Verification items for the finished model (mm, model axes). A direction names the side the tool comes from. Coordinates: 2 decimals unless noted, no trailing zeros. Order: outer loops, then holes, each group sorted by start corner. A loop starts at its lowest first (then second) coordinate and runs counter-clockwise, first axis right, second up. Notation, with made-up numbers: (-4.5, 71) -> (49.5, 71) arc R18 cw to (49.5, 82) -> close; hole circle Ø5 at (-28, 74). An arc over 180 degrees is marked (long way). Write item = value, one per line. Start each with the question number.
1. Set-up check for faces 1 (the flat face through (9, 0, -2)), 2 (the flat face through (4.04, 0, -3)), 3 (the flat face through (-8, 0, -2)): record each of +Z, -Z, +X, -X, +Y, -Y from which the full face is reachable in a straight line by a thin tool's end or side.
2. Thickness scan on line 1 along X through (y, z) = (0.85, -4.25); line 2 along X through (y, z) = (0.5, -1); line 3 along Z through (x, y) = (1.5, 0.05). Record the ranges inside material, lowest first. Write a range as from..to.
3. Cross-section at A-A on z = -3.25. Record the cut outline in (x, y), plus the area to 3 significant figures.
4. Cross-section at D-D on x = -1. Record the cut outline in (y, z), plus the area to 3 significant figures.
5. Cross-section at B-B on y = -0.3. Record the cut outline in (x, z), plus the area to 3 significant figures.
6. Cross-section at C-C on z = -1.25. Record the cut outline in (x, y), plus the area to 3 significant figures.
7. Go/stop test with flat-tipped pins: P1, Ø3, axis at x = 9, y = 1, coming from the +Z side; P2, Ø1.8, axis at y = 0.5, z = 3, coming from the +X side; P3, Ø2, axis at y = 1, z = 2.5, coming from the -X side. Record where each tip stops, or that it passes through.
8. Release check for a two-part mould opening along X. For faces 4 (the flat face through (0, 0, 8.59)), 5 (the flat face through (-3.56, 0, -3)), 6 (the flat face through (10.04, 0, -4)) record: +X half, -X half, draft (parallel to the pull), parting line (faces both ways), or undercut.
from build123d import *

# Parameters (mm, degrees)
SKETCH1_W           = 14.5
SKETCH1_H           = 5.9
BOSS_EXTRUDE1_DEPTH = 2.59
SKETCH2_W           = 3.689926182
SKETCH2_H           = 5.9
SKETCH2_W_2         = 3.210073818
BOSS_EXTRUDE2_DEPTH = 2
SKETCH5_W           = 6
SKETCH5_H           = 5.9
BOSS_EXTRUDE3_DEPTH = 4
SKETCH7_W           = 14.5
SKETCH7_H           = 5.9
BOSS_EXTRUDE5_DEPTH = 6
FILLET2_R           = 1


with BuildPart() as part:
    # Sketch1 → Boss-Extrude1 (new body)
    with BuildSketch(Plane.XY):
        Rectangle(SKETCH1_W, SKETCH1_H)
    extrude(amount=BOSS_EXTRUDE1_DEPTH)

    # Sketch2 → Boss-Extrude2 (add)
    with BuildSketch(Plane(origin=(0, 0, 0), x_dir=(-1, 0, 0), z_dir=(0, 0, -1))):
        with Locations((5.405036909, 0)):
            Rectangle(SKETCH2_W, SKETCH2_H)
        with Locations((-5.644963091, 0)):
            Rectangle(SKETCH2_W_2, SKETCH2_H)
    extrude(amount=BOSS_EXTRUDE2_DEPTH)

    # Sketch5 → Boss-Extrude3 (add)
    with BuildSketch(Plane(origin=(0, 0, -2), x_dir=(-1, 0, 0), z_dir=(0, 0, -1))):
        with Locations((-7.039926182, 0)):
            Rectangle(SKETCH5_W, SKETCH5_H)
        with Locations((6.560073818, 0)):
            Rectangle(SKETCH5_W, SKETCH5_H)
    extrude(amount=BOSS_EXTRUDE3_DEPTH)

    # Sketch7 → Boss-Extrude5 (add)
    with BuildSketch(Plane.XY.offset(2.59)):
        Rectangle(SKETCH7_W, SKETCH7_H)
    extrude(amount=BOSS_EXTRUDE5_DEPTH)

    # Fillet2
    fillet2_edges = [part.edges().sort_by_distance(p)[0] for p in [
        (0, 2.95, 8.59),
        (-7.25, 0, 8.59),
        (0, -2.95, 8.59),
        (7.25, 0, 8.59),
    ]]
    fillet(fillet2_edges, radius=FILLET2_R)


solid = part.part
Worked out:
q1.face_1 = +Z, +X, +Y, -Y
q1.face_2 = -Z, +Y, -Y
q1.face_3 = +Z, -X, +Y, -Y
q2.line_1 = -9.56..-3.56, 4.04..10.04
q2.line_2 = -7.25..-3.56, 4.04..7.25
q2.line_3 = 0..8.59
q3.outline = (-9.56, -2.95) -> (-3.56, -2.95) -> (-3.56, 2.95) -> (-9.56, 2.95) -> close; (4.04, -2.95) -> (10.04, -2.95) -> (10.04, 2.95) -> (4.04, 2.95) -> close
q3.area = 70.8 mm²
q4.outline = (-2.95, 0) -> (2.95, 0) -> (2.95, 7.59) arc R1 ccw to (1.95, 8.59) -> (-1.95, 8.59) arc R1 ccw to (-2.95, 7.59) -> close
q4.area = 50.3 mm²
q5.outline = (-9.56, -6) -> (-3.56, -6) -> (-3.56, 0) -> (4.04, 0) -> (4.04, -6) -> (10.04, -6) -> (10.04, -2) -> (7.25, -2) -> (7.25, 7.59) arc R1 ccw to (6.25, 8.59) -> (-6.25, 8.59) arc R1 ccw to (-7.25, 7.59) -> (-7.25, -2) -> (-9.56, -2) -> close
q5.area = 186 mm²
q6.outline = (-7.25, -2.95) -> (-3.56, -2.95) -> (-3.56, 2.95) -> (-7.25, 2.95) -> close; (4.04, -2.95) -> (7.25, -2.95) -> (7.25, 2.95) -> (4.04, 2.95) -> close
q6.area = 40.7 mm²
q7.P1 = -2
q7.P2 = 7.25
q7.P3 = -7.25
q8.face_4 = draft
q8.face_5 = undercut
q8.face_6 = +X half
